Autodesk Inventor part; units mm, degrees
ref_plane "YZ Plane" through (0, 0, 0) normal (1, 0, 0) x (0, 1, 0)
ref_plane "XZ Plane" through (0, 0, 0) normal (0, 1, 0) x (-1, 0, 0)
ref_plane "XY Plane" through (0, 0, 0) normal (0, 0, 1) x (1, 0, 0)
sketch "Sketch1" plane through (0, 0, 0) normal (0, 1, 0) x (-1, 0, 0)
  circle A0 centre (0, 0) radius 4
  dimension "d0" = 8
extrude "Extrusion1" add sketch "Sketch1" along normal blind 20
sketch "Sketch2" plane through (0, 20, 0) normal (0, 1, 0) x (1, 0, 0)
  circle A0 centre (0, 0) radius 3
  dimension "d3" = 6
extrude "Extrusion2" add sketch "Sketch2" along normal blind 15
fillet "Fillet1" radius 2 1 edges at (4, 20, 0)
sketch "Sketch3" plane through (0, 35, 0) normal (0, 1, 0) x (1, 0, 0)
  circle A0 centre (0, 0) radius 1.5
  dimension "d7" = 3
extrude "Extrusion3" cut sketch "Sketch3" against normal blind 35
CAD build for the part. Positions are in the model's coordinates, mm. Round coordinates to 2 decimals unless told otherwise and drop trailing zeros. Order: outer loops, then holes, each group sorted by start corner. A loop starts at its lowest first (then second) coordinate and runs counter-clockwise, first axis right, second up. Notation, with made-up numbers: (37.25, 29) - (62.25, 29) arc R22 ccw to (62.25, 58) - close; hole circle Ø10 at (46.25, 27.25). An arc over 180 degrees is marked (long way). Use CSV: the item, a comma, the result in double quotes. Start each with the question number.
1) Pin check, flat tips, straight feed: pin 1 Ø1.5 at (x, z) = (-0.5, 3) entering from +Y; pin 2 Ø2 at (x, y) = (-1.5, 20) entering from -Z. Stop position of each tip, or through.
2) Two-plate mould, pull along Z, no slides. Class faces 1 (the cylindrical face through (-3, 27, 0)), 2 (the cylindrical face through (-1.5, 17.74, -0.07)), 3 (the flat face through (1.3, 35, 1.3)): pulls with the +Z half, pulls with the -Z half, needs draft (parallel to the pull), parting line crosses it, or undercut.
3) Saw through at A-A (y = 4). List the corners of the cut face in (x, z).
4) Saw through at B-B (y = 22). List the corners of the cut face in (x, z), and give its area (3 significant figures).
5) Wall check: L1, parallel to X at y = 29.5, z = 0; L2, parallel to Z at x = 0, y = 15. Give the ranges that are in metal, low to high. Write a range as [from, to].
Values follow:
1,pin 1,"stops at y = 35"
1,pin 2,"stops at z = -3.67"
2,face 1,"parting line crosses it"
2,face 2,"undercut"
2,face 3,"needs draft"
3,outline,"circle Ø8 at (0, 0); hole circle Ø3 at (0, 0)"
4,outline,"circle Ø6 at (0, 0); hole circle Ø3 at (0, 0)"
4,area,"21.2 mm2"
5,L1,"x = [-3, -1.5], [1.5, 3]"
5,L2,"z = [-4, -1.5], [1.5, 4]"
